Source: CAD feature listing. Evaluate the final solid. Frame: model axes, mm. A direction names the side the tool comes from. Round coordinates to 2 decimals unless told otherwise and drop trailing zeros. Order: outer loops, then holes, each group sorted by start corner. A loop starts at its lowest first (then second) coordinate and runs counter-clockwise, first axis right, second up. Notation, with made-up numbers: (11.5, 17) -> (46.5, 17) arc R25 cw to (46.5, 39) -> close; hole circle Ø9 at (31.5, -21). An arc over 180 degrees is marked (long way). One line per item, written item: value. Start each with the question number.
1) Pin query (flat end, axial travel): P1, Ø4, axis at x = 12.7, z = -14.29, coming from the -Y side; P2, Ø8, axis at x = 19.5, z = -12, coming from the +Y side; P3, Ø4, axis at x = 12, y = 18, coming from the +Z side; P4, Ø3, axis at x = 3, y = 21.5, coming from the -Z side (3 decimals). Return the tip coordinate at first contact, or that it passes through.
2) Section D-D (x = 19.5). Return the cut outline in (y, z) (3 decimals), and give its area (3 significant figures).
3) Mould query, pull axis Y, two halves, no side actions, for faces 3 (the face through (1.29, 1.61, -24.15)), 4 (the face through (1.29, 24.15, -1.57)), 5 (the face through (12.369, 16.806, -1.565)). Classes: pulls with the +Y half, pulls with the -Y half, needs draft (parallel to the pull), parting line crosses it, or undercut.
4) Section A-A (x = 12.7). Return the cut outline in (y, z) (1 decimal), and give its area (3 significant figures).
5) Section C-C (z = -14). Return the cut outline in (x, y) (3 decimals).
6) Section B-B (y = 13.5). Return the cut outline in (x, z) (3 decimals), and give its area (3 significant figures).
7) Ray query, L1, parallel to Y at x = 12.7, z = -1.25; L2, parallel to Z at x = 23, y = 14.5 (3 decimals); L3, parallel to Y at x = 3.5, z = -17.25 (3 decimals). Return the intervals inside material, ascending.
8) Reachability of faces 1 (the face through (13, 0, -10)), 2 (the face through (13, 3.175, -19)) from +Z, -Z, +X, -X, +Y, -Y: full face, straight path, thin tool, end or side. Return the list, or none.
```python
from build123d import *

# Parameters (mm, degrees)
BOSS_EXTRUDE1_DEPTH = 25.4
SKETCH2_R           = 2.54
CUT_EXTRUDE1_DEPTH  = 44.994090512
SKETCH3_R           = 2.54
CUT_EXTRUDE2_DEPTH  = 44.994090512
FILLET1_R           = 5.08
CHAMFER1_SIZE       = 2.54


with BuildPart() as part:
    # Sketch1 → Boss-Extrude1 (new body)
    with BuildSketch(Plane(origin=(0, 0, 0), x_dir=(0, 0, -1), z_dir=(1, 0, 0))):
        Polygon((0, 0), (0, 25.4), (3.175, 25.4), (3.175, 3.175), (25.4, 3.175), (25.4, 0), align=None)
    extrude(amount=BOSS_EXTRUDE1_DEPTH)

    # Sketch2 → Cut-Extrude1 (cut, through all)
    with BuildSketch(Plane.XY):
        with Locations((12.7, 14.2875)):
            Circle(SKETCH2_R)
    extrude(amount=-CUT_EXTRUDE1_DEPTH, mode=Mode.SUBTRACT)

    # Sketch3 → Cut-Extrude2 (cut, through all)
    with BuildSketch(Plane.XZ):
        with Locations(Location((12.7, -14.2875, 0), (0, 0, 270))):
            Circle(SKETCH3_R)
    extrude(amount=-CUT_EXTRUDE2_DEPTH, mode=Mode.SUBTRACT)

    # Fillet1
    fillet1_edges = [part.edges().sort_by_distance(p)[0] for p in [
        (12.7, 3.175, -3.175),
    ]]
    fillet(fillet1_edges, radius=FILLET1_R)

    # Chamfer1
    chamfer1_edges = [part.edges().sort_by_distance(p)[0] for p in [
        (25.4, 25.4, -1.5875),
        (0, 25.4, -1.5875),
        (0, 1.5875, -25.4),
        (25.4, 1.5875, -25.4),
    ]]
    chamfer(chamfer1_edges, length=CHAMFER1_SIZE)


solid = part.part
```
Findings:
1. P1: through
1. P2: y = 3.18
1. P3: z = 0
1. P4: z = -3.175
2. outline: (0, -25.4) -> (3.175, -25.4) -> (3.175, -8.255) arc R5.08 cw to (8.255, -3.175) -> (25.4, -3.175) -> (25.4, 0) -> (0, 0) -> close
2. area: 157 mm2
3. face 3: needs draft
3. face 4: pulls with the +Y half
3. face 5: undercut
4. outline: (0, -25.4) -> (3.2, -25.4) -> (3.2, -16.8) -> (0, -16.8) -> close; (0, -11.7) -> (3.2, -11.7) -> (3.2, -8.3) arc R5.1 cw to (8.3, -3.2) -> (11.7, -3.2) -> (11.7, 0) -> (0, 0) -> close; (16.8, -3.2) -> (25.4, -3.2) -> (25.4, 0) -> (16.8, 0) -> close
4. area: 124 mm2
5. outline: (0, 0) -> (10.176, 0) -> (10.176, 3.175) -> (0, 3.175) -> close; (15.224, 0) -> (25.4, 0) -> (25.4, 3.175) -> (15.224, 3.175) -> close
6. outline: (0, -3.175) -> (10.285, -3.175) -> (10.285, 0) -> (0, 0) -> close; (15.115, -3.175) -> (25.4, -3.175) -> (25.4, 0) -> (15.115, 0) -> close
6. area: 65.3 mm2
7. L1: 0 to 11.75, 16.83 to 25.4
7. L2: -3.175 to 0
7. L3: 0 to 3.175
8. face 1: +Z, -Z, +X, -X, -Y
8. face 2: -Z, +X, -X, +Y
